Read the model definition and answer for the solid it produces. Units are mm, in the model's axes. A direction names the side the tool comes from. Coordinates: 2 decimals unless noted, no trailing zeros. Loops run counter-clockwise (first coordinate to the right, second up) from the corner with the lowest first, then second, coordinate; pieces in that order, holes last.
from build123d import *

# Parameters (mm, degrees)
F0_W         = 147
F0_H         = 60
F1_DEPTH     = 3
F2_W         = 3
F2_H         = 60
F3_DEPTH     = 20
F4_DEPTH     = 4
F5_W         = 141
F5_H         = 4
F6_DEPTH     = 20
F7_DEPTH     = 2
F8_DEPTH     = 2
F10_W        = 5
F10_H        = 11.305693537
F11_DEPTH    = 15
F9_R         = 1.25
F12_DEPTH    = 25
F13_T4_DEPTH = 82.150489639
F13_T9_DEPTH = 82.150489639
F14_W        = 14.2459415197
F14_H        = 3
F14_W_2      = 46.2986054569
F14_W_3      = 5
F14_W_4      = 78.4554530233
F15_DEPTH    = 25
F16_SIZE     = 25
F17_W        = 109.1084168532
F17_H        = 3
F18_DEPTH    = 25
F19_W        = 67.5222836435
F19_H        = 44.9108928442
F19_W_2      = 29.4727757573
F19_H_2      = 45.0668334961
F20_DEPTH    = 25
F21_W        = 65.4478734359
F21_H        = 13.5871618986
F22_DEPTH    = 25
F23_W        = 46.1584180593
F23_H        = 4
F24_DEPTH    = 25


# Not quite as in the source:
# - a fillet or chamfer that OpenCascade refuses, or shapes differently, is made with other operations: its cross-section is extruded or revolved along the edge and cut away or added


with BuildPart() as f1:
    # F0 (on Front) → F1 (new body)
    with BuildSketch(Plane.XZ):
        with Locations((39.3571183681, 3.4620302916)):
            Rectangle(F0_W, F0_H)
    extrude(amount=F1_DEPTH)

    # F2 (on face) → F3 (join)
    with BuildSketch(Plane.XZ.offset(3)):
        with Locations((-32.6428816319, 3.4620302916)):
            Rectangle(F2_W, F2_H)
        with Locations((111.3571183681, 3.4620302916)):
            Rectangle(F2_W, F2_H)
    extrude(amount=F3_DEPTH)

    # F4 (add): a face of the model
    f4_faces = [f1.faces().sort_by_distance(p)[0] for p in [
        (-32.6549972277, -11.5, -26.5379697084),
    ]]
    extrude(f4_faces, amount=F4_DEPTH)

    # F5 (on face) → F6 (join)
    with BuildSketch(Plane.XZ.offset(3)):
        with Locations((39.3571183681, -28.5379697084)):
            Rectangle(F5_W, F5_H)
    extrude(amount=F6_DEPTH)

    # F7 (add): a face of the model
    f7_faces = [f1.faces().sort_by_distance(p)[0] for p in [
        (112.8571183681, -11.5, 1.4620302916),
    ]]
    extrude(f7_faces, amount=F7_DEPTH)

    # F8 (cut): a face of the model
    f8_faces = [f1.faces().sort_by_distance(p)[0] for p in [
        (109.8571183681, -13, 3.4620302916),
    ]]
    extrude(f8_faces, amount=-F8_DEPTH, mode=Mode.SUBTRACT)

    # F10 (on face) → F11 (join)
    with BuildSketch(Plane(origin=(0, 0, -30.5379697084), x_dir=(1, 0, 0), z_dir=(0, 0, -1))):
        with Locations((-17.3969401121, 5.6528467685)):
            Rectangle(F10_W, F10_H)
        with Locations((66.0585129112, 5.6528467685)):
            Rectangle(F10_W, F10_H)
    extrude(amount=F11_DEPTH)

    # F9 (on face) → F12 (cut)
    with BuildSketch(Plane.XZ.offset(3)):
        with Locations((-16.1428816319, 4.912131466)):
            Circle(F9_R)
        with Locations((68.8571183681, 4.912131466)):
            Circle(F9_R)
    extrude(amount=-F12_DEPTH, mode=Mode.SUBTRACT)

    # F13: chamfer of 15 on 2 edges, made by hand


with BuildPart() as f13_tool2:
    # F13_s3 → F13_t4 (new body)
    with BuildSketch(Plane.YZ.offset(23.6783047074)):
        Polygon((3.694306463, -45.5379697084), (-11.305693537, -30.5379697084), (-11.305693537, -45.5379697084), align=None)
    extrude(amount=-F13_T4_DEPTH)

    split(bisect_by=Plane.XY.offset(-30.5379697084), keep=Keep.BOTTOM)


with BuildPart() as f1_1:
    add(f1.part)

    # F13_t1: cut F13_tool2
    add(f13_tool2.part, mode=Mode.SUBTRACT)


with BuildPart() as f13_tool7:
    # F13_s8 → F13_t9 (new body)
    with BuildSketch(Plane.YZ.offset(107.1337577307)):
        Polygon((3.694306463, -45.5379697084), (-11.305693537, -30.5379697084), (-11.305693537, -45.5379697084), align=None)
    extrude(amount=-F13_T9_DEPTH)

    split(bisect_by=Plane.XY.offset(-30.5379697084), keep=Keep.BOTTOM)


with BuildPart() as f1_2:
    add(f1_1.part)

    # F13_t6: cut F13_tool7
    add(f13_tool7.part, mode=Mode.SUBTRACT)

    # F14 (on face) → F15 (join)
    with BuildSketch(Plane(origin=(0, 0, -30.5379697084), x_dir=(1, 0, 0), z_dir=(0, 0, -1))):
        with Locations((-27.019910872, 1.5)):
            Rectangle(F14_W, F14_H)
        with Locations((91.7078156397, 1.5)):
            Rectangle(F14_W_2, F14_H)
        with Locations((-17.3969401121, 1.5)):
            Rectangle(F14_W_3, F14_H)
        with Locations((66.0585129112, 1.5)):
            Rectangle(F14_W_3, F14_H)
        with Locations((24.3307863995, 1.5)):
            Rectangle(F14_W_4, F14_H)
    extrude(amount=F15_DEPTH)

    # F16
    f16_edges = [f1_2.edges().sort_by_distance(p)[0] for p in [
        (114.857118, -1.5, -55.53797),
    ]]
    chamfer(f16_edges, length=F16_SIZE)

    # F17 (on face) → F18 (join)
    with BuildSketch(Plane.XZ.offset(3)):
        with Locations((20.4113267948, -54.0379697084)):
            Rectangle(F17_W, F17_H)
    extrude(amount=F18_DEPTH)

    # F19 (on face) → F20 (cut)
    with BuildSketch(Plane.XZ.offset(3)):
        with Locations((27.5696460158, 3.6646034569)):
            Rectangle(F19_W, F19_H)
        with Locations((90.4137082398, 3.7425737828)):
            Rectangle(F19_W_2, F19_H_2)
    extrude(amount=-F20_DEPTH, mode=Mode.SUBTRACT)

    # F21 (on face) → F22 (cut)
    with BuildSketch(Plane.XZ.offset(3)):
        with Locations((27.9176128097, -41.5276624262)):
            Rectangle(F21_W, F21_H)
    extrude(amount=-F22_DEPTH, mode=Mode.SUBTRACT)

    # F23 (on face) → F24 (join)
    with BuildSketch(Plane.XZ.offset(23)):
        with Locations((34.9768251181, -28.5379697084)):
            Rectangle(F23_W, F23_H)
    extrude(amount=F24_DEPTH)


solid = f1_2.part
Item 1: A cutting plane is placed at D-D on x = 92. Determine the outline of the cut face in (y, z).
Numbers:
outline: (-23, -30.54) - (-3, -30.54) - (-3, -53.4) - (0, -53.4) - (0, -18.79) - (-3, -18.79) - (-3, -26.54) - (-23, -26.54) - close; (-3, 26.28) - (0, 26.28) - (0, 33.46) - (-3, 33.46) - close
Item 2: Given pin 1 (4 mm diameter, centred on x = 69.5, y = -22.5, fed in from +Z); pin 2 (12.5 mm diameter, centred on x = 65.5, z = -48, fed in from -Y); pin 3 (2.5 mm diameter, centred on y = -6.5, z = -36, fed in from -X), each flat-ended and moving along its own axis, determine where each tip first touches the part or whether it passes through.
Numbers:
pin 1: stops at z = -26.54
pin 2: stops at y = -28
pin 3: stops at x = -19.9
Item 3: A cutting plane is placed at C-C on z = 23. Determine the outline of the cut face in (x, y).
Numbers:
outline: (-34.14, -23) - (-31.14, -23) - (-31.14, -3) - (-6.19, -3) - (-6.19, 0) - (-34.14, 0) - close; (61.33, -3) - (75.68, -3) - (75.68, 0) - (61.33, 0) - close; (105.15, -3) - (111.86, -3) - (111.86, -23) - (114.86, -23) - (114.86, 0) - (105.15, 0) - close
Item 4: A cutting plane is placed at B-B on x = -3. Determine the outline of the cut face in (y, z).
Numbers:
outline: (-28, -55.54) - (0, -55.54) - (0, -48.32) - (-3, -48.32) - (-3, -52.54) - (-28, -52.54) - close; (-23, -30.54) - (-3, -30.54) - (-3, -34.73) - (0, -34.73) - (0, -18.79) - (-3, -18.79) - (-3, -26.54) - (-23, -26.54) - close; (-3, 26.12) - (0, 26.12) - (0, 33.46) - (-3, 33.46) - close
Item 5: Determine the mould class of faces 1 (the face through (114.857, -11, 2)), 2 (the face through (60.642, -2, -42)), 3 (the face through (23, -2, 33.462)), 4 (the face through (-6.191, -2, 3)) for opening direction Z: released by +Z, released by -Z, zero draft, split by the parting line, or undercut.
Numbers:
face 1: zero draft
face 2: undercut
face 3: released by +Z
face 4: undercut
Item 6: Which of the six approach directions +Z, -Z, +X, -X, +Y, -Y give full straight-line access (tool end or side, diameter ignored) to faces 5 (the face through (39, -20, -30.538)), 6 (the face through (58.056, -35, -29)), 7 (the face through (66.094, -7.095, -34.749))?
Numbers:
face 5: -Y
face 6: +Z, +X, -Y
face 7: +X, -X, -Y
Item 7: A cutting plane is placed at A-A on y = -19. Determine the outline of the cut face in (x, z), then the cut area to 3 significant figures.
Numbers:
outline: (-34.14, -55.54) - (74.97, -55.54) - (74.97, -52.54) - (-34.14, -52.54) - close; (-34.14, -30.54) - (114.86, -30.54) - (114.86, 33.46) - (111.86, 33.46) - (111.86, -26.54) - (-31.14, -26.54) - (-31.14, 33.46) - (-34.14, 33.46) - close
area: 1,280 mm2
Item 8: Find the intervals of material crossed by line 1 along Z through (x, y) = (-27.5, -7); line 2 along X through (y, z) = (-15.5, -25); line 3 along Y through (x, z) = (49, -20), in increasing order.
Numbers:
line 1: z = -55.54 to -52.54, -30.54 to -26.54
line 2: x = -34.14 to -31.14, 111.86 to 114.86
line 3: y = -3 to 0
